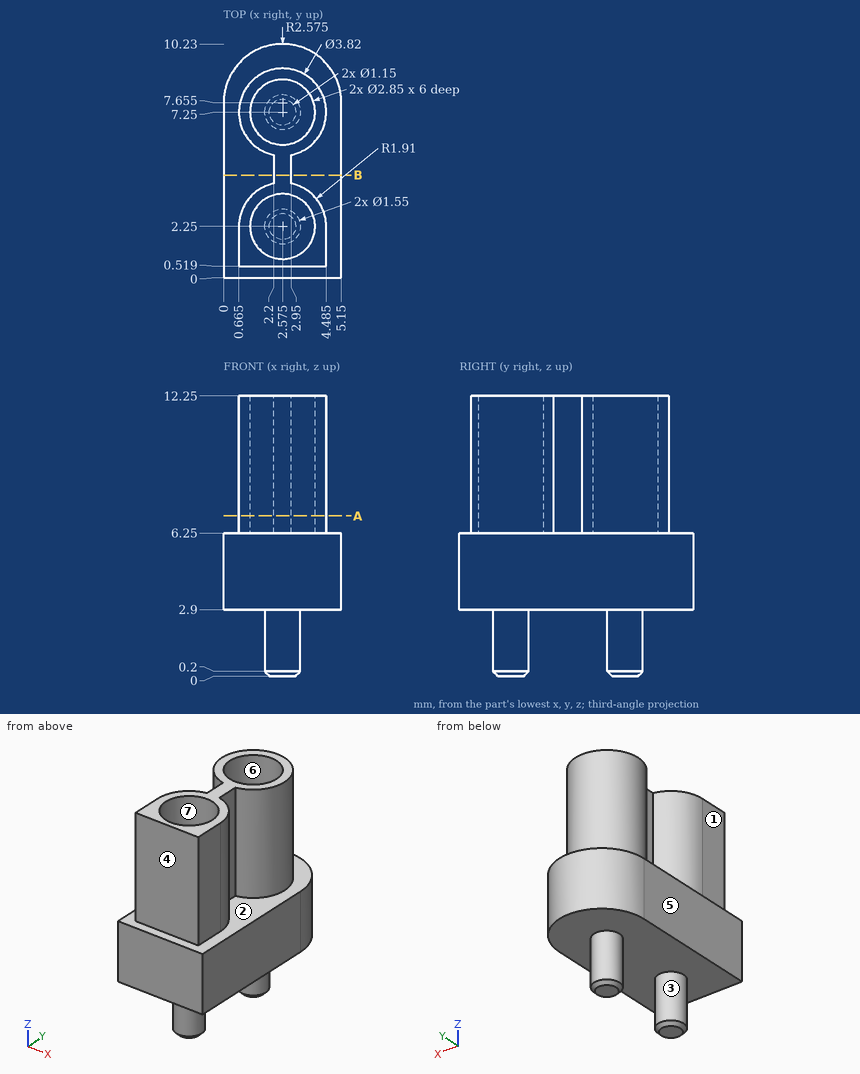
Study the drawing (mm; zero at the part's minimum x, y, z) and answer. A direction names the side the tool comes from. Round coordinates to 2 decimals unless told otherwise and drop trailing zeros. Write each loop counter-clockwise with the first axis right and the second up, starting at its lowest first coordinate (ties: lowest second). Pieces come first, ordered by that corner, then holes.
Q1. The mould has two halves that part along X. Classify the marked faces 4, 5, 6 and 7: released by +X, released by -X, zero draft, split by the parting line, or undercut.
Values:
face 4: zero draft
face 5: released by -X
face 6: undercut
face 7: undercut
Q2. Flat-ended cylindrical pins translate along their axes: P1, Ø1.9, axis at x = 3.5, z = 9.5, coming from the -Y side; P2, Ø1.9, axis at y = 1, z = 9, coming from the +X side (3 decimals); P3, Ø1.9, axis at y = 1.5, z = 8.5, coming from the -X side (3 decimals). Find the tip coordinate at first contact, or state that the pin passes through.
Values:
P1: stops at y = 0.52
P2: stops at x = 4.485
P3: stops at x = 0.665
Q3. A tool of negligible diameter and unlimited length cuts with its end or side. For the marked faces 1, 2 and 3, from which of +Z, -Z, +X, -X, +Y, -Y can it reach the whole face along a straight path? Write none if from no direction.
Values:
face 1: +Z, -X, +Y, -Y
face 2: +Z
face 3: -Z
Q4. Find section A-A on z = 7. State how many separate pieces and enclosed holes the cut face has.
Values:
separate pieces: 1
enclosed holes: 2
Q5. Straight lines are drawn through the part: line 1 (Z direction, x = 2.4, y = 7); line 2 (Z direction, x = 2.5, y = 1); line 3 (X direction, y = 7.75, z = 9.75). For each, find the intervals that lie inside material, in ascending order.
Values:
line 1: z = 0 to 6.25
line 2: z = 2.9 to 6.25
line 3: x = 0.73 to 1.24, 3.91 to 4.42
Q6. Find section B-B on y = 4.5. Determine the outline of the cut face in (x, z).
Values:
outline: (0, 2.9) - (5.15, 2.9) - (5.15, 6.25) - (2.95, 6.25) - (2.95, 12.25) - (2.2, 12.25) - (2.2, 6.25) - (0, 6.25) - close
